Can you work these out from the model? Positions are in its coordinate system, mm. Round coordinates to 2 decimals unless told otherwise and drop trailing zeros. Order: outer loops, then holes, each group sorted by start corner. A loop starts at its lowest first (then second) coordinate and runs counter-clockwise, first axis right, second up. Notation, with made-up numbers: (80, -7.75) -> (131, -7.75) arc R22 cw to (131, 15.25) -> close; hole circle Ø6 at (44, 74.25). An arc over 180 degrees is marked (long way). Use a Markdown table: item, result. Add a question column.
Q1. I need wall thicknesses on line 1 along Y through (x, z) = (212, -8); line 2 along Y through (x, z) = (224, -4.75); line 3 along X through (y, z) = (152, -6.5). Which ranges of each line are inside material? Lowest first, please. Write a range as [from, to].
Q2. If we section it at A-A on y = -140: List the corners of the cut face in (x, z) for me, plus the area to 3 significant figures.
Q3. I'm going to push flat-ended pins straight in: pin 1 Ø6 at (x, z) = (224, 4.5) entering from +Y; pin 2 Ø6 at (y, z) = (148.5, -1.5) entering from -X. Where does each tip first touch, or does it pass through?
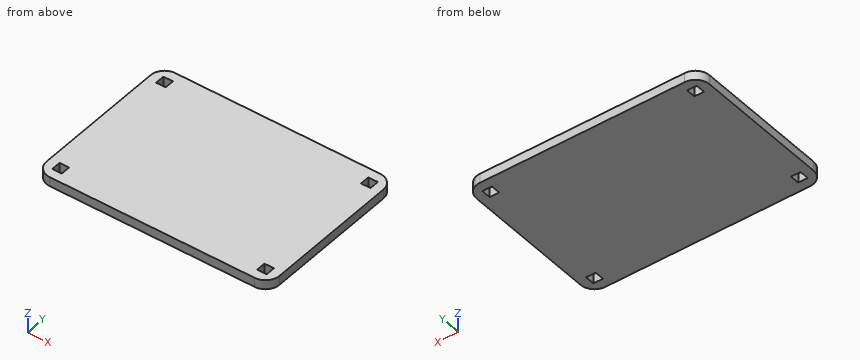
Autodesk Inventor part; units mm, degrees
sketch "Esboço1" plane through (0, 0, 0) normal (0, 0, 1) x (1, 0, 0)
  line L0 (-250, -175) -> (250, -175)
  line L1 (250, -175) -> (250, 175)
  line L2 (250, 175) -> (-250, 175)
  line L3 (-250, 175) -> (-250, -175)
  line L4 (-250, -175) -> (250, 175) construction
  line L5 (250, -175) -> (-250, 175) construction
  point P0 (0, 0)
  dimension "d0" = 500
  dimension "d1" = 350
extrude "Extrusão1" add sketch "Esboço1" along normal mid plane 20
fillet "Arredondamento1" radius 30 4 edges at (-250, 175, 0) (250, 175, 0) (250, -175, 0) (-250, -175, 0)
sketch "Esboço2" plane through (0, 0, 10) normal (0, 0, 1) x (1, 0, 0)
  line L0 (230, 135) -> (230, 155)
  line L1 (230, 155) -> (210, 155)
  line L2 (210, 155) -> (210, 135)
  line L3 (210, 135) -> (230, 135)
  line L4 (212, 137) -> (212, 153)
  line L5 (212, 153) -> (228, 153)
  line L6 (228, 153) -> (228, 137)
  line L7 (228, 137) -> (212, 137)
  line L8 (209.8, 155.2) -> (230.2, 155.2)
  line L9 (230.2, 155.2) -> (230.2, 134.8)
  line L10 (230.2, 134.8) -> (209.8, 134.8)
  line L11 (209.8, 134.8) -> (209.8, 155.2)
  line L12 (-210, 135) -> (-210, 155)
  line L13 (-210, 155) -> (-230, 155)
  line L14 (-230, 155) -> (-230, 135)
  line L15 (-230, 135) -> (-210, 135)
  line L16 (-228, 137) -> (-228, 153)
  line L17 (-228, 153) -> (-212, 153)
  line L18 (-212, 153) -> (-212, 137)
  line L19 (-212, 137) -> (-228, 137)
  line L20 (-210, -155) -> (-210, -135)
  line L21 (-210, -135) -> (-230, -135)
  line L22 (-230, -135) -> (-230, -155)
  line L23 (-230, -155) -> (-210, -155)
  line L24 (-228, -153) -> (-228, -137)
  line L25 (-228, -137) -> (-212, -137)
  line L26 (-212, -137) -> (-212, -153)
  line L27 (-212, -153) -> (-228, -153)
  line L28 (230, -135) -> (230, -155)
  line L29 (230, -155) -> (210, -155)
  line L30 (210, -155) -> (210, -135)
  line L31 (210, -135) -> (230, -135)
  line L32 (212, -137) -> (212, -153)
  line L33 (212, -153) -> (228, -153)
  line L34 (228, -153) -> (228, -137)
  line L35 (228, -137) -> (212, -137)
  line L36 (-230.2, 155.2) -> (-209.8, 155.2)
  line L37 (-209.8, 155.2) -> (-209.8, 134.8)
  line L38 (-209.8, 134.8) -> (-230.2, 134.8)
  line L39 (-230.2, 134.8) -> (-230.2, 155.2)
  line L40 (-230.2, -134.8) -> (-209.8, -134.8)
  line L41 (-209.8, -134.8) -> (-209.8, -155.2)
  line L42 (-209.8, -155.2) -> (-230.2, -155.2)
  line L43 (-230.2, -155.2) -> (-230.2, -134.8)
  line L44 (230.2, -155.2) -> (230.2, -134.8)
  line L45 (230.2, -134.8) -> (209.8, -134.8)
  line L46 (209.8, -134.8) -> (209.8, -155.2)
  line L47 (209.8, -155.2) -> (230.2, -155.2)
  point P0 (0, 0)
  dimension "d5" = 0.2
  dimension "d6" = 0.2
  dimension "d7" = 0.2
  dimension "d8" = 0.2
extrude "Extrusão2" cut sketch "Esboço2" against normal blind 20 contours L3 L2 L1 L0 | L4 L5 L6 L7 | L8 L9 L10 L11 | L15 L14 L13 L12 | L16 L17 L18 L19 | L23 L22 L21 L20 | L24 L25 L26 L27 | L28 L29 L30 L31 | L35 L34 L33 L32 | L36 L37 L38 L39 | L40 L41 L42 L43 | L47 L46 L45 L44
properties part number "Sessao8_07_04_2025_0001_0001" material "Ouro"
Answer below:
| question | item | result |
|---|---|---|
| 1 | line 1 | [-175, -155.2], [-134.8, 134.8], [155.2, 175] |
| 1 | line 2 | [-174.73, -155.2], [-134.8, 134.8], [155.2, 174.73] |
| 1 | line 3 | [-249.17, -230.2], [-209.8, 209.8], [230.2, 249.17] |
| 2 | outline | (-250, -10) -> (-230.2, -10) -> (-230.2, 10) -> (-250, 10) -> close; (-209.8, -10) -> (209.8, -10) -> (209.8, 10) -> (-209.8, 10) -> close; (230.2, -10) -> (250, -10) -> (250, 10) -> (230.2, 10) -> close |
| 2 | area | 9,180 mm² |
| 3 | pin 1 | y = 174.98 |
| 3 | pin 2 | x = -250 |
